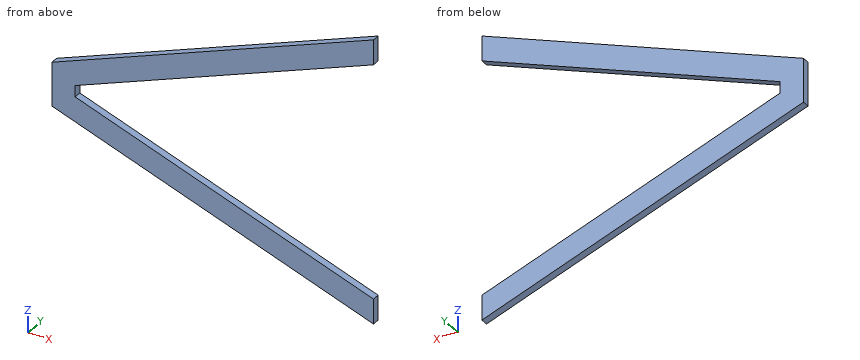
Autodesk Inventor part; units mm, degrees
ref_plane "YZ Plane" through (0, 0, 0) normal (1, 0, 0) x (0, 1, 0)
ref_plane "XZ Plane" through (0, 0, 0) normal (0, 1, 0) x (-1, 0, 0)
ref_plane "XY Plane" through (0, 0, 0) normal (0, 0, 1) x (1, 0, 0)
sketch "Sketch1" plane through (0, 0, 0) normal (0, 1, 0) x (-1, 0, 0)
  line L0 (0, 0) -> (0, -10.16)
  line L1 (0, -10.16) -> (166.6875, -72.0318)
  line L2 (166.6875, -72.0318) -> (170.0021, -63.1021)
  line L3 (170.0021, -63.1021) -> (0, 0)
  line L4 (0, -133.9036) -> (166.6875, -72.0318)
  line L5 (170.0021, -80.9615) -> (0, -144.0636)
  line L6 (0, -144.0636) -> (0, -133.9036)
  line L7 (166.6875, -72.0318) -> (170.0021, -80.9615)
  line L8 (170.0021, -63.1021) -> (160.4771, -63.1021)
  line L9 (160.4771, -63.1021) -> (160.4771, -80.9615)
  line L10 (160.4771, -80.9615) -> (170.0021, -80.9615)
  line L11 (170.0021, -80.9615) -> (170.0021, -63.1021)
  line L12 (0, 0) -> (38.1, 0)
  line L13 (38.1, 0) -> (38.1, -144.0636)
  line L14 (38.1, -144.0636) -> (0, -144.0636)
  line L15 (0, -144.0636) -> (0, 0)
  point P0 (160.4771, -69.7266)
  point P1 (160.4771, -74.337)
  dimension "d0" = 10.16
  dimension "d1" = 9.525
  dimension "d2" = 177.8
  dimension "d3" = 177.8
  dimension "d4" = 10.16
  dimension "d5" = 9.525
  dimension "d6" = 9.525
  dimension "d9" = 38.1
extrude "Extrusion1" add sketch "Sketch1" along normal blind 3.175 contours L3 L13 L1 L0 | L3 L8 L9 L1 L13 | L4 L13 L5 L6 | L11 L7 L2 | L2 L1 L9 L8 | L1 L4 L9 | L4 L9 L10 L5 L13 | L7 L10 L9 L4
sketch "Sketch2" plane through (0, 3.175, 0) normal (0, 1, 0) x (1, 0, 0)
  line L0 (0, 0) -> (0, 10.16)
  line L1 (0, 0) -> (-38.1, 0)
  line L2 (-38.1, 0) -> (-38.1, 144.0636)
  line L3 (-38.1, 144.0636) -> (0, 144.0636)
  line L4 (0, 144.0636) -> (0, 0)
  dimension "d10" = 38.1
extrude "Extrusion2" cut sketch "Sketch2" against normal blind 3.175
properties part number "Projectile Launcher Back" material "Wood (Birch)"
Can you work these out from the model? Positions are in its coordinate system, mm. Give positions to 0.01 mm unless a question says otherwise; leave off trailing zeros. Order: outer loops, then holes, each group sorted by start corner. A loop starts at its lowest first (then second) coordinate and runs counter-clockwise, first axis right, second up. Notation, with made-up numbers: M 0.25,58.25 L 6.25,58.25 A29 cw 6.25,89.25 Z; hole C -21,83.5 d9. An arc over 180 degrees is marked long. Write item = value, one per line. Start each with the question number.
Q1. Suppose I cut it at B-B (x = -115). Write out the boundary of the cut face in (y, z) (3 decimals), plus the area to 3 significant figures.
Q2. Will these pins go through, and if not, where does the flat tip stop? pin 1 Ø2 at (x, z) = (-96, -110.5) entering from -Y; pin 2 Ø1 at (y, z) = (1.5, -72) entering from +X.
Q3. Suppose I cut it at D-D (z = -52.5). Write out the boundary of the cut face in (x, y) (3 decimals).
Q4. I need wall thicknesses on probe 1 along Z at (x, y) = (-112, 1.15); probe 2 along Z at (x, y) = (-150.5, 2.9); probe 3 along X at (y, z) = (0.2, -70). Which ranges of each line are inside material? Lowest first, please. Write a range as [from, to].
Q5. Suppose I cut it at C-C (z = -66.5). Write out the boundary of the cut face in (x, y) (3 decimals), plus the area to 3 significant figures.
Q6. Suppose I cut it at A-A (y = 1.9). Write out the boundary of the cut face in (x, z).
Check result:
q1.outline = M 0,-101.377 L 3.175,-101.377 L 3.175,-91.217 L 0,-91.217 Z; M 0,-52.846 L 3.175,-52.846 L 3.175,-42.686 L 0,-42.686 Z
q1.area = 64.5 mm2
q2.pin_1 = through
q2.pin_2 = -160.48
q3.outline = M -141.439,0 L -114.067,0 L -114.067,3.175 L -141.439,3.175 Z
q4.probe_1 = [-102.49, -92.33], [-51.73, -41.57]
q4.probe_2 = [-88.2, -78.04], [-66.02, -55.86]
q4.probe_3 = [-170, -160.48]
q5.outline = M -170.002,0 L -151.784,0 L -151.784,3.175 L -170.002,3.175 Z
q5.area = 57.8 mm2
q6.outline = M -170,-80.96 L -38.1,-129.92 L -38.1,-119.76 L -160.48,-74.34 L -160.48,-69.73 L -38.1,-24.3 L -38.1,-14.14 L -170,-63.1 Z
